Input: part model. Units: mm. Frame: model coordinates. Face numbers are marked on the shaded views. A direction names the side the tool comes from. Coordinates: 2 decimals unless noted, no trailing zeros. Order: outer loops, then holes, each group sorted by start corner. A loop starts at its lowest first (then second) coordinate and runs counter-clockwise, first axis right, second up. Notation, with made-up numbers: (18, 17.5) - (53, 17.5) arc R16 ccw to (53, 28.5) - close; hole circle Ø3 at (37.5, -40). An arc over 180 degrees is marked (long way). Answer as CSV lines item,"result". Start each with the question number.
Item 1: Section B-B (x = 5). Output: boundary loops of the cut face in (y, z), and give its area (3 significant figures).
Item 2: Access query for the marked faces 4, 5 and 6. Directions: +Z, -Z, +X, -X, +Y, -Y. A direction counts if a zero-diameter tool reaches every point of the face in a straight line with its end or side. Return the directions, or none.
Item 3: Section C-C (y = 13). Output: boundary loops of the cut face in (x, z).
Item 4: Section A-A (z = 16). Output: boundary loops of the cut face in (x, y), and give its area (3 significant figures).
Item 5: First-contact query: pin 1 (8 mm diameter, centred on y = 5.5, z = -11.5, fed in from -X). Flat tip, straight axial feed; report the tip coordinate or a pass-through.
Item 6: Draft query along X for the marked faces 1, 2 and 3. Return one class per face: +X half, -X half, draft (parallel to the pull), parting line (faces both ways), or undercut.
Item 7: Section D-D (y = 31). Output: boundary loops of the cut face in (x, z), and give its area (3 significant figures).
Item 8: Material intervals for line 1 along Z through (x, y) = (-0.1, 30.9); line 2 along Y through (x, z) = (9.5, 3); line 3 along Y through (x, z) = (12, 15.5), sorted ascending.
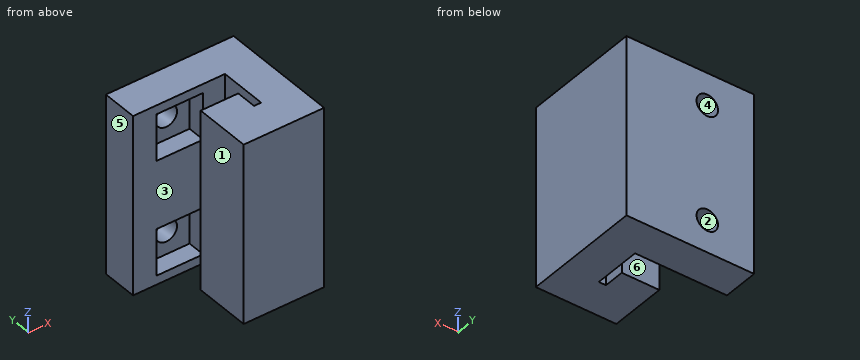
from build123d import *

# Parameters (mm, degrees)
F1_DEPTH = 25
F2_R     = 3
F3_DEPTH = 10
F4_W     = 13
F4_H     = 13
F5_DEPTH = 5


with BuildPart() as f1:
    # F0 (on Top) → F1 (new body, symmetric)
    with BuildSketch(Plane.XY):
        Polygon((22.5, 0), (22.5, 33.3), (-13.2, 33.3), (-13.2, 23.3), (12.5, 23.3), (12.5, 10), (10.5, 10), (10.5, 15.8), (0, 15.8), (0, 0), align=None)
    extrude(amount=F1_DEPTH, both=True)

    # F2 (on face) → F3 (cut, through all)
    with BuildSketch(Plane(origin=(0, 33.3, 0), x_dir=(-1, 0, 0), z_dir=(0, 1, 0))):
        with Locations((0.1, -16)):
            Circle(F2_R)
        with Locations((0.1, 16)):
            Circle(F2_R)
    extrude(amount=-F3_DEPTH, mode=Mode.SUBTRACT)

    # F4 (on face) → F5 (cut)
    with BuildSketch(Plane.XZ.offset(-23.3)):
        with Locations((-0.1, 16)):
            Rectangle(F4_W, F4_H)
        with Locations((-0.1, -16)):
            Rectangle(F4_W, F4_H)
    extrude(amount=-F5_DEPTH, mode=Mode.SUBTRACT)


solid = f1.part
Determined:
1,outline,"(0, -25) - (15.8, -25) - (15.8, 25) - (0, 25) - close; (23.3, -25) - (33.3, -25) - (33.3, 25) - (23.3, 25) - (23.3, 22.5) - (28.3, 22.5) - (28.3, 9.5) - (23.3, 9.5) - (23.3, -9.5) - (28.3, -9.5) - (28.3, -22.5) - (23.3, -22.5) - close"
1,area,"1,160 mm^2"
2,face 4,"+Y"
2,face 5,"+Z, -Z, -X, +Y, -Y"
2,face 6,"+Z, -Z, -X"
3,outline,"(0, -25) - (10.5, -25) - (10.5, 25) - (0, 25) - close; (12.5, -25) - (22.5, -25) - (22.5, 25) - (12.5, 25) - close"
4,outline,"(-13.2, 23.3) - (-6.6, 23.3) - (-6.6, 28.3) - (-3.1, 28.3) - (-3.1, 33.3) - (-13.2, 33.3) - close; (0, 0) - (22.5, 0) - (22.5, 33.3) - (2.9, 33.3) - (2.9, 28.3) - (6.4, 28.3) - (6.4, 23.3) - (12.5, 23.3) - (12.5, 10) - (10.5, 10) - (10.5, 15.8) - (0, 15.8) - close"
4,area,"681 mm^2"
5,pin 1,"stops at x = 0"
6,face 1,"-X half"
6,face 2,"undercut"
6,face 3,"draft"
7,outline,"(-13.2, -25) - (22.5, -25) - (22.5, 25) - (-13.2, 25) - close; hole circle Ø6 at (-0.1, -16); hole circle Ø6 at (-0.1, 16)"
7,area,"1,730 mm^2"
8,line 1,"z = -25 to -19, -13 to 13, 19 to 25"
8,line 2,"y = 0 to 15.8, 23.3 to 33.3"
8,line 3,"y = 0 to 10, 23.3 to 33.3"
